```python
from build123d import *

# Parameters (mm, degrees)
F0_W     = 50
F0_H     = 60
F1_DEPTH = 6
F2_W     = 6
F2_H     = 60
F3_DEPTH = 44
F5_DEPTH = 50.001
F6_R     = 2.25
F6_R_2   = 3.3
F7_DEPTH = 25


with BuildPart() as f1:
    # F0 (on Top) → F1 (new body)
    with BuildSketch(Plane.XY):
        with Locations((25, -30)):
            Rectangle(F0_W, F0_H)
    extrude(amount=F1_DEPTH)

    # F2 (on face) → F3 (join)
    with BuildSketch(Plane.XY.offset(6)):
        with Locations((3, -30)):
            Rectangle(F2_W, F2_H)
    extrude(amount=F3_DEPTH)

    # F4 (on face) → F5 (cut, through all)
    with BuildSketch(Plane(origin=(0, 0, 0), x_dir=(0, -1, 0), z_dir=(-1, 0, 0))):
        with BuildLine():
            Line((50, 29.25), (35, 29.25))
            ThreePointArc((35, 29.25), (32.75, 27), (35, 24.75))
            Line((35, 24.75), (50, 24.75))
            ThreePointArc((50, 24.75), (52.25, 27), (50, 29.25))
        make_face()
    extrude(amount=-F5_DEPTH, mode=Mode.SUBTRACT)

    # F6 (on face) → F7 (cut)
    with BuildSketch(Plane.XY.offset(6)):
        with Locations((27.5, -30)):
            Circle(F6_R)
        with Locations((15, -30)):
            Circle(F6_R_2)
        with Locations((40, -30)):
            Circle(F6_R_2)
    extrude(amount=-F7_DEPTH, mode=Mode.SUBTRACT)


solid = f1.part
```
Can you work these out from the model? Positions are in its coordinate system, mm. A direction names the side the tool comes from. Coordinates: 2 decimals unless noted, no trailing zeros. Order: outer loops, then holes, each group sorted by start corner. A loop starts at its lowest first (then second) coordinate and runs counter-clockwise, first axis right, second up.
1. Thinking about a two-plate mould opening in Y: for faces 4 (the face through (5, -60, 14)), 5 (the face through (33, -30, 6)), 6 (the face through (28.538, -31.996, 3.042)), which applies, +Y half, -Y half, draft (parallel to the pull), parting line (faces both ways), or undercut?
2. If we section it at B-B (y = -39): Please give me the cut outline in (x, z), then the cut area to 3 significant figures.
3. If we section it at A-A (z = 27): Please give me the cut outline in (x, y), then the cut area to 3 significant figures.
4. If we section it at C-C (z = 4): Please give me the cut outline in (x, y).
5. If we section it at D-D (x = 41): Please give me the cut outline in (y, z), then the cut area to 3 significant figures.
6. For faces 1 (the face through (3, -42, 24.75)), 2 (the face through (25, -30, 0)), 3 (the face through (6, -30, 28)), which set-ups out of +Z, -Z, +X, -X, +Y, -Y let a thin tool reach every point of the face, with its end or its side?
7. I'm going to push flat-ended pins straight in: pin 1 (10 mm diameter, centred on y = -29, z = 28, fed in from +X); pin 2 (2.5 mm diameter, centred on x = 27.5, y = -30, fed in from +Z). Where does each tip first touch, or does it pass through?
8. I need wall thicknesses on line 1 (Z direction, x = 2, y = -45); line 2 (Y direction, x = 40, z = 2.9); line 3 (Z direction, x = 19, y = -40). Which ranges of each line are inside material? Lowest first, please.
Entries:
1. face 4: -Y half
1. face 5: draft
1. face 6: undercut
2. outline: (0, 0) - (50, 0) - (50, 6) - (6, 6) - (6, 24.75) - (0, 24.75) - close; (0, 29.25) - (6, 29.25) - (6, 50) - (0, 50) - close
2. area: 537 mm2
3. outline: (0, -60) - (6, -60) - (6, -52.25) - (0, -52.25) - close; (0, -32.75) - (6, -32.75) - (6, 0) - (0, 0) - close
3. area: 243 mm2
4. outline: (0, -60) - (50, -60) - (50, 0) - (0, 0) - close; hole circle Ø6.6 at (15, -30); hole circle Ø4.5 at (27.5, -30); hole circle Ø6.6 at (40, -30)
5. outline: (-60, 0) - (-33.14, 0) - (-33.14, 6) - (-60, 6) - close; (-26.86, 0) - (0, 0) - (0, 6) - (-26.86, 6) - close
5. area: 322 mm2
6. face 1: +X, -X
6. face 2: -Z, +X, -X, +Y, -Y
6. face 3: +Z, +X, +Y, -Y
7. pin 1: stops at x = 6
7. pin 2: passes through
8. line 1: z = 0 to 24.75, 29.25 to 50
8. line 2: y = -60 to -33.3, -26.7 to 0
8. line 3: z = 0 to 6
